Study the drawing (mm; zero at the part's minimum x, y, z) and answer. A direction names the side the tool comes from. Coordinates: 2 decimals unless noted, no trailing zeros. Loops run counter-clockwise (first coordinate to the right, second up) from the corner with the lowest first, then second, coordinate; pieces in that order, holes last. Notation, with made-up numbers: (27, -38.75) - (43, -38.75) arc R19 ccw to (43, -17.75) - close; hole circle Ø4 at (0.25, 34). An arc over 180 degrees is marked (long way). Use one line per item in the form item = value.
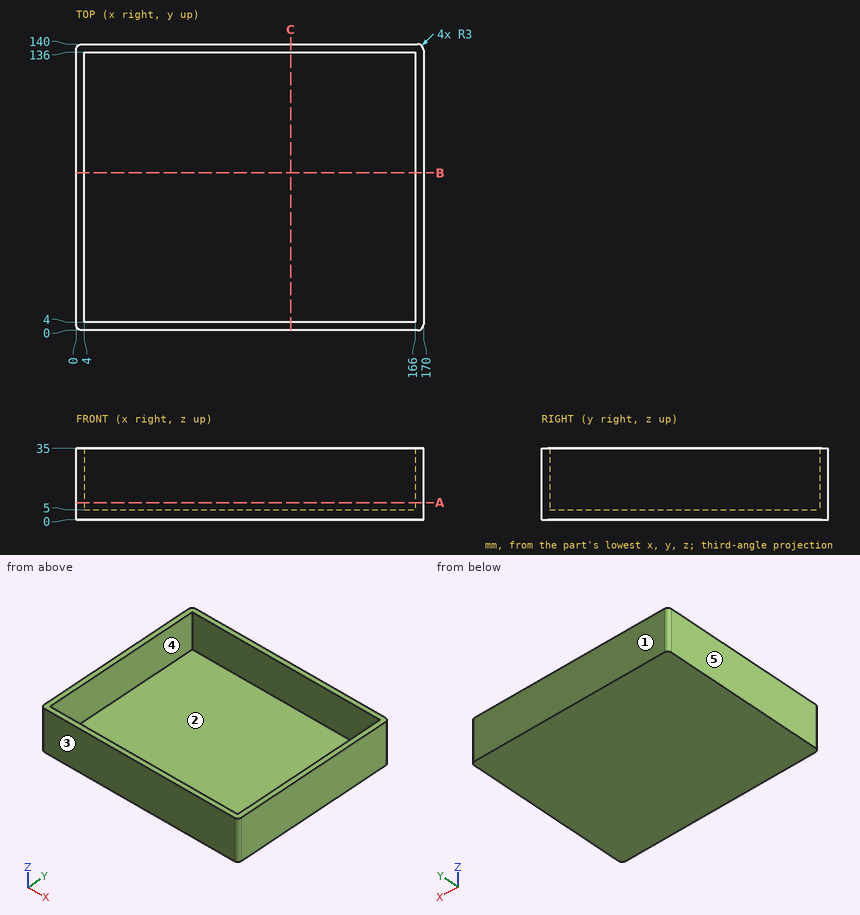
Item 1: For a pull along X with two mould halves and no side action, classify the marked faces 3, 4 and 5 as +X half, -X half, draft (parallel to the pull), parting line (faces both ways), or undercut.
Results below:
face_3 = draft
face_4 = undercut
face_5 = -X half
Item 2: This flat-tipped pin is pushed along its axis until it touches: P1, Ø1.5, axis at x = 43.5, y = 61, coming from the +Z side. Where does it stop, or does it pass through?
Results below:
P1 = 5
Item 3: The part is cut by section A-A on z = 8.5. Give the vertices of the cut face in (x, y), plus the area to 3 significant figures.
Results below:
outline = (0, 3) arc R3 ccw to (3, 0) - (167, 0) arc R3 ccw to (170, 3) - (170, 137) arc R3 ccw to (167, 140) - (3, 140) arc R3 ccw to (0, 137) - close; hole (4, 4) - (166, 4) - (166, 136) - (4, 136) - close
area = 2,410 mm²
Item 4: Find the intervals of material crossed by L1, parallel to X at y = 61, z = 26.5; L2, parallel to Y at x = 129, z = 33; L3, parallel to Z at x = 111, y = 125.5, in increasing order.
Results below:
L1 = 0 to 4, 166 to 170
L2 = 0 to 4, 136 to 140
L3 = 0 to 5
Item 5: Which of the six approach directions +Z, -Z, +X, -X, +Y, -Y give full straight-line access (tool end or side, diameter ignored) to the marked faces 1 and 2?
Results below:
face_1 = +Z, -Z, +X, -X, +Y
face_2 = +Z
Item 6: The part is cut by section B-B on y = 77. Give the vertices of the cut face in (x, z), plus the area to 3 significant figures.
Results below:
outline = (0, 0) - (170, 0) - (170, 35) - (166, 35) - (166, 5) - (4, 5) - (4, 35) - (0, 35) - close
area = 1,090 mm²
Item 7: The part is cut by section C-C on x = 105. Give the vertices of the cut face in (y, z), plus the area to 3 significant figures.
Results below:
outline = (0, 0) - (140, 0) - (140, 35) - (136, 35) - (136, 5) - (4, 5) - (4, 35) - (0, 35) - close
area = 940 mm²
